Geometry: see drawing. Coordinates: mm, zero at the bounding-box minimum. A direction names the side the tool comes from. Round coordinates to 2 decimals unless told otherwise and drop trailing zeros. Order: outer loops, then holes, each group sorted by start corner. A loop starts at its lowest first (then second) coordinate and runs counter-clockwise, first axis right, second up.
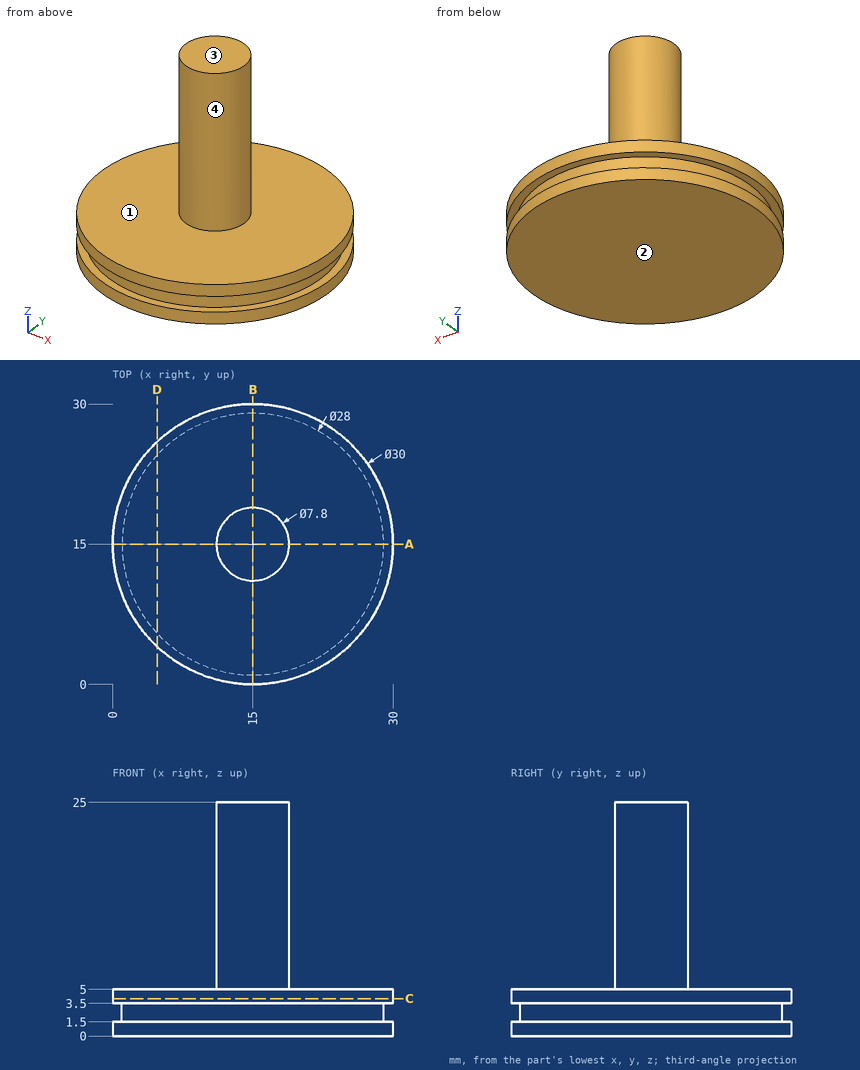
1. Pull-direction query (X, two-part tool) for the marked faces 3 and 4; classes: released by +X, released by -X, zero draft, split by the parting line, or undercut.
2. Section C-C on z = 4. Return loops of the section in (x, y).
3. Section A-A on y = 15. Return loops of the section in (x, z).
4. Access query for the marked faces 1 and 2. Directions: +Z, -Z, +X, -X, +Y, -Y. A direction counts if a zero-diameter tool reaches every point of the face in a straight line with its end or side. Return the directions, or none.
5. Section D-D on x = 4.75. Return loops of the section in (y, z), plus the area to 3 significant figures.
6. First-contact query: pin 1 (12 mm diameter, centred on x = 3, y = 23, fed in from +Z); pin 2 (9 mm diameter, centred on x = 17.5, y = 19.5, fed in from +Z); pin 3 (12 mm diameter, centred on y = 11, z = 19.5, fed in from -X); pin 4 (3 mm diameter, centred on x = 9, z = 9.5, fed in from -Y). Flat tips, straight axial feed; report the tip coordinate or a pass-through.
7. Line query: line 1 along Z through (x, y) = (28.25, 21.25); line 2 along Z through (x, y) = (14, 20); line 3 along Y through (x, z) = (12.75, 9). Output: solid intervals per line, ascending.
Result:
1. face 3: zero draft
1. face 4: split by the parting line
2. outline: circle Ø30 at (15, 15)
3. outline: (0, 0) - (30, 0) - (30, 1.5) - (29, 1.5) - (29, 3.5) - (30, 3.5) - (30, 5) - (18.9, 5) - (18.9, 25) - (11.1, 25) - (11.1, 5) - (0, 5) - (0, 3.5) - (1, 3.5) - (1, 1.5) - (0, 1.5) - close
4. face 1: +Z
4. face 2: -Z, +X, -X, +Y, -Y
5. outline: (4.05, 0) - (25.95, 0) - (25.95, 1.5) - (24.54, 1.5) - (24.54, 3.5) - (25.95, 3.5) - (25.95, 5) - (4.05, 5) - (4.05, 3.5) - (5.46, 3.5) - (5.46, 1.5) - (4.05, 1.5) - close
5. area: 104 mm2
6. pin 1: stops at z = 5
6. pin 2: stops at z = 25
6. pin 3: stops at x = 11.1
6. pin 4: passes through
7. line 1: z = 0 to 1.5, 3.5 to 5
7. line 2: z = 0 to 5
7. line 3: y = 11.81 to 18.19
